```python
from build123d import *

# Parameters (mm, degrees)
CUT_EXTRUDE1_DEPTH      = 46.738386504
CUT_EXTRUDE1_DEPTH_BACK = 46.738386504
SKETCH2_R               = 3
CHAMFER1_SIZE           = 1
SKETCH3_W               = 1.55
SKETCH3_H               = 1.5
CUT_EXTRUDE3_START      = -1
SKETCH4_R               = 14.7
SKETCH4_R_2             = 11.05
CUT_EXTRUDE3_DEPTH      = 1
SKETCH5_W               = 2
SKETCH5_H               = 3
SKETCH5_W_2             = 3
SKETCH5_H_2             = 2
CUT_EXTRUDE4_DEPTH      = 15
FILLET1_R               = 1
CHAMFER2_SIZE           = 2


with BuildPart() as part:
    # Sketch1 → Revolve1 (revolve)
    with BuildSketch(Plane.XY, mode=Mode.PRIVATE) as revolve1_sk:
        Polygon((0, 0), (11.05, 0), (11.05, 15), (18, 15), (18, 20), (8, 20), (8, 38), (0, 38), align=None)
    revolve(revolve1_sk.sketch.rotate(Axis((0, 0, 0), (0, 1, 0)), 90), axis=Axis((0, 0, 0), (0, 1, 0)))

    # Sketch2 → Cut-Extrude1 (cut, two sides: drawn at the far end of the back side and taken through both)
    with BuildSketch(Plane.XY.offset(-CUT_EXTRUDE1_DEPTH_BACK)):
        with Locations((0, 30.7)):
            Circle(SKETCH2_R)
    extrude(amount=CUT_EXTRUDE1_DEPTH + CUT_EXTRUDE1_DEPTH_BACK, mode=Mode.SUBTRACT)

    # Chamfer1
    chamfer1_edges = [part.edges().sort_by_distance(p)[0] for p in [
        (0, 15, 18),
    ]]
    chamfer(chamfer1_edges, length=CHAMFER1_SIZE)

    # Sketch3 → Cut-Revolve1 (revolve, cut)
    with BuildSketch(Plane.XY, mode=Mode.PRIVATE) as cut_revolve1_sk:
        with Locations((10.275, 2.25)):
            Rectangle(SKETCH3_W, SKETCH3_H)
        with Locations((10.275, 5.25)):
            Rectangle(SKETCH3_W, SKETCH3_H)
        with Locations((10.275, 8.25)):
            Rectangle(SKETCH3_W, SKETCH3_H)
        with Locations((10.275, 11.25)):
            Rectangle(SKETCH3_W, SKETCH3_H)
        with Locations((10.275, 14.25)):
            Rectangle(SKETCH3_W, SKETCH3_H)
    revolve(cut_revolve1_sk.sketch.rotate(Axis((0, -2, 0), (0, 1, 0)), 90), axis=Axis((0, -2, 0), (0, 1, 0)), mode=Mode.SUBTRACT)

    # Sketch4 → Cut-Extrude3 (cut)
    with BuildSketch(Plane.XZ.offset(-15).offset(CUT_EXTRUDE3_START)):
        with Locations(Location((0, 0, 0), (0, 0, 270))):
            Circle(SKETCH4_R)
        with Locations(Location((0, 0, 0), (0, 0, 270))):
            Circle(SKETCH4_R_2, mode=Mode.SUBTRACT)
    extrude(amount=CUT_EXTRUDE3_DEPTH, mode=Mode.SUBTRACT)

    # Sketch5 → Cut-Extrude4 (cut)
    with BuildSketch(Plane.XZ):
        with Locations((0, -10.5)):
            Rectangle(SKETCH5_W, SKETCH5_H)
        with Locations((0, 10.5)):
            Rectangle(SKETCH5_W, SKETCH5_H)
        with Locations((-10.5, 0)):
            Rectangle(SKETCH5_W_2, SKETCH5_H_2)
        with Locations((10.5, 0)):
            Rectangle(SKETCH5_W_2, SKETCH5_H_2)
    extrude(amount=-CUT_EXTRUDE4_DEPTH, mode=Mode.SUBTRACT)

    # Fillet1
    fillet1_edges = [part.edges().sort_by_distance(p)[0] for p in [
        (9.223610907, 15, -1),
        (9.223610907, 15, 1),
        (-1, 15, -9.223610907),
        (1, 15, -9.223610907),
        (-9.223610907, 15, 1),
        (-9.223610907, 15, -1),
        (1, 15, 9.223610907),
        (-1, 15, 9.223610907),
    ]]
    fillet(fillet1_edges, radius=FILLET1_R - 0.0001)  # a hair under: the kernel refuses the full size

    # Chamfer2
    chamfer2_edges = [part.edges().sort_by_distance(p)[0] for p in [
        (0, 38, 8),
    ]]
    chamfer(chamfer2_edges, length=CHAMFER2_SIZE)


solid = part.part
```
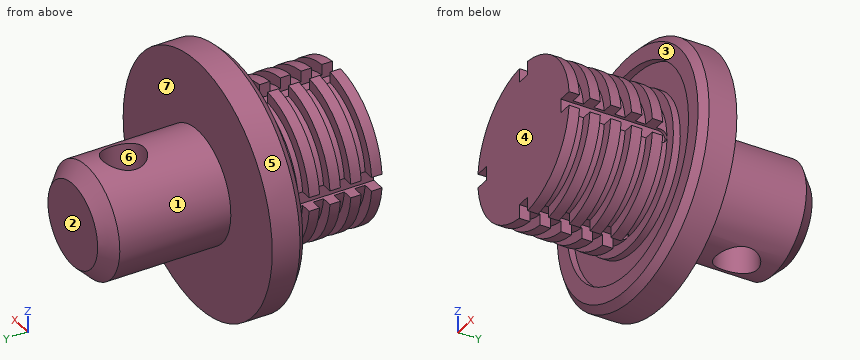
Geometry check sheet. Reference: the model listing, model coordinates, mm. Face numbers are marked on the shaded views. A direction names the side the tool comes from. Coordinates: 2 decimals unless noted, no trailing zeros. Loops run counter-clockwise (first coordinate to the right, second up) from the corner with the lowest first, then second, coordinate; pieces in that order, holes last.
Item 1: Thickness scan on line 1 (Y direction, x = -4.5, z = 9); line 2 (Y direction, x = 0, z = 1.75); line 3 (X direction, y = 15.85, z = 0). Record the ranges inside material, lowest first.
Item 2: Access from +Z, -Z, +X, -X, +Y, -Y to the whole of each face (thin tool, end or side, straight path). Record for the marked faces 1, 2 and 3.
Item 3: Release check for a two-part mould opening along Y. For the marked faces 4, 5, 6 and 7 record: released by +Y, released by -Y, zero draft, split by the parting line, or undercut.
Item 4: Sectioned sample at A-A, the plane y = 21.5. Record the boundary of the cut face in (x, z), then the cut area to 3 significant figures.
Item 5: Sectioned sample at C-C, the plane y = 17. Record the boundary of the cut face in (x, z).
Item 6: Go/stop test with flat-tipped pins: pin 1 Ø5 at (y, z) = (11.5, 5.5) entering from -X; pin 2 Ø7 at (x, y) = (0, 30.7) entering from -Z; pin 3 Ø8 at (x, z) = (-6.5, -7) entering from +Y; pin 4 Ø1.5 at (x, z) = (7.5, -10) entering from +Y. Record where each tip stops, or that it passes through.
Item 7: Sectioned sample at B-B, the plane y = 29. Record the boundary of the cut face in (x, z).
Check result:
1. line 1: y = 0 to 1.5, 3 to 4.5, 6 to 7.5, 9 to 10.5, 12 to 13.5, 15 to 20
1. line 2: y = 0 to 27.7, 33.7 to 38
1. line 3: x = -17.85 to -14.7, -11.05 to 11.05, 14.7 to 17.85
2. face 1: +Y
2. face 2: +Z, -Z, +X, -X, +Y
2. face 3: -Y
3. face 4: released by -Y
3. face 5: zero draft
3. face 6: undercut
3. face 7: released by +Y
4. outline: circle Ø16 at (0, 0)
4. area: 201 mm2
5. outline: circle Ø36 at (0, 0)
6. pin 1: stops at x = -10.62
6. pin 2: stops at z = -8
6. pin 3: stops at y = 38
6. pin 4: stops at y = 20
7. outline: (-2.47, -7.61) - (-2.47, 7.61) arc R8 ccw to start; (2.47, -7.61) arc R8 ccw to (2.47, 7.61) - close
